```python
from build123d import *

# Parameters (mm, degrees)
SKETCH2_R           = 3.5
SKETCH2_R_2         = 1.5
BOSS_EXTRUDE1_DEPTH = 3.5
FILLET1_R           = 10
SKETCH3_R           = 1
CUT_EXTRUDE1_DEPTH  = 10


with BuildPart() as part:
    # Sketch2 → Boss-Extrude1 (new body)
    with BuildSketch(Plane.XY):
        with BuildLine():
            Line((-56.161165235, -8.838834765), (0, 47.32233047))
            Line((0, 47.32233047), (56.161165235, -8.838834765))
            ThreePointArc((56.161165235, -8.838834765), (73.838834765, -8.838834765), (73.838834765, 8.838834765))
            Line((73.838834765, 8.838834765), (0, 82.67766953))
            Line((0, 82.67766953), (-73.838834765, 8.838834765))
            ThreePointArc((-73.838834765, 8.838834765), (-73.838834765, -8.838834765), (-56.161165235, -8.838834765))
        make_face()
        with Locations((-65, 0)):
            Circle(SKETCH2_R, mode=Mode.SUBTRACT)
        with Locations((65, 0)):
            Circle(SKETCH2_R, mode=Mode.SUBTRACT)
        with Locations((0, 65)):
            Circle(SKETCH2_R_2, mode=Mode.SUBTRACT)
    extrude(amount=-BOSS_EXTRUDE1_DEPTH)

    # Fillet1
    fillet1_edges = [part.edges().sort_by_distance(p)[0] for p in [
        (0, 82.67766953, -1.75),
        (0, 47.32233047, -1.75),
    ]]
    fillet(fillet1_edges, radius=FILLET1_R)

    # Sketch3 → Cut-Extrude1 (cut)
    with BuildSketch(Plane.XY):
        with Locations((-52.625631329, 27.223611076)):
            Circle(SKETCH3_R)
        with Locations((-37.776388924, 12.374368671)):
            Circle(SKETCH3_R)
        with Locations((37.776388924, 12.374368671)):
            Circle(SKETCH3_R)
        with Locations((52.625631329, 27.223611076)):
            Circle(SKETCH3_R)
    extrude(amount=-CUT_EXTRUDE1_DEPTH, mode=Mode.SUBTRACT)


solid = part.part
```
Check sheet for the modelled part. Datum: model origin and axes. Units: mm. A direction names the side the tool comes from. Round coordinates to 2 decimals unless told otherwise and drop trailing zeros. Write each loop counter-clockwise with the first axis right and the second up, starting at its lowest first coordinate (ties: lowest second). Pieces come first, ordered by that corner, then holes. Notation, with made-up numbers: (31.25, 55) -> (64.25, 55) arc R9 cw to (64.25, 60) -> close; hole circle Ø3 at (-17, -14). An arc over 180 degrees is marked (long way). One line per question, with ' | ' between items. Start each with the question number.
1. Sectioned sample at C-C, the plane y = 0. Record the cut outline in (x, z), then the cut area to 3 significant figures.
2. Sectioned sample at A-A, the plane x = 0. Record the cut outline in (y, z), then the cut area to 3 significant figures.
3. Sectioned sample at D-D, the plane z = -2.5. Record the cut outline in (x, y), then the cut area to 3 significant figures.
4. Release check for a two-part mould opening along X. For faces 1 (the face through (11, 40, -3.5)), 2 (the face through (-0.11, 78.535, -1.774)), 3 (the face through (0.806, 66.265, -1.726)), 4 (the face through (-39.99, 42.69, -1.73)) record: +X half, -X half, draft (parallel to the pull), parting line (faces both ways), or undercut.
5. Scan lines: line 1 along X through (y, z) = (2, -2.8); line 2 along X through (y, z) = (-2, -2.45); line 3 along X through (y, z) = (19, -1). Record each from-to range of solid material in increasing order. Write a range as from..to.
6. Sectioned sample at B-B, the plane y = 65. Record the cut outline in (x, z), then the cut area to 3 significant figures.
7. Depth check by flat-ended pin: pin 1 (1 mm diameter, centred on y = 66, z = -2, fed in from +X); pin 2 (2 mm diameter, centred on y = 58.5, z = -1, fed in from +X); pin 3 (1.5 mm diameter, centred on y = 62, z = -0.5, fed in from +X). Enter the tip coordinate at first touch or a pass-through.
8. Set-up check for faces 5 (the face through (11, 40, 0)), 6 (the face through (-31.96, 15.36, -1.73)): record each of +Z, -Z, +X, -X, +Y, -Y from which the full face is reachable in a straight line by a thin tool's end or side.
Taken from the geometry:
1) outline: (-77.5, -3.5) -> (-68.5, -3.5) -> (-68.5, 0) -> (-77.5, 0) -> close; (-61.5, -3.5) -> (-47.32, -3.5) -> (-47.32, 0) -> (-61.5, 0) -> close; (47.32, -3.5) -> (61.5, -3.5) -> (61.5, 0) -> (47.32, 0) -> close; (68.5, -3.5) -> (77.5, -3.5) -> (77.5, 0) -> (68.5, 0) -> close | area: 162 mm^2
2) outline: (43.18, -3.5) -> (63.5, -3.5) -> (63.5, 0) -> (43.18, 0) -> close; (66.5, -3.5) -> (78.54, -3.5) -> (78.54, 0) -> (66.5, 0) -> close | area: 113 mm^2
3) outline: (-73.84, 8.84) arc R12.5 ccw to (-56.16, -8.84) -> (-7.07, 40.25) arc R10 cw to (7.07, 40.25) -> (56.16, -8.84) arc R12.5 ccw to (73.84, 8.84) -> (7.07, 75.61) arc R10 ccw to (-7.07, 75.61) -> close; hole circle Ø7 at (-65, 0); hole circle Ø2 at (-52.63, 27.22); hole circle Ø2 at (-37.78, 12.37); hole circle Ø3 at (0, 65); hole circle Ø2 at (37.78, 12.37); hole circle Ø2 at (52.63, 27.22); hole circle Ø7 at (65, 0) | area: 4,990 mm^2
4) face 1: draft | face 2: parting line | face 3: undercut | face 4: -X half
5) line 1: x = -77.34..-67.87, -62.13..-45.32, 45.32..62.13, 67.87..77.34 | line 2: x = -77.34..-67.87, -62.13..-49.32, 49.32..62.13, 67.87..77.34 | line 3: x = -63.68..-28.32, 28.32..63.68
6) outline: (-17.68, -3.5) -> (-1.5, -3.5) -> (-1.5, 0) -> (-17.68, 0) -> close; (1.5, -3.5) -> (17.68, -3.5) -> (17.68, 0) -> (1.5, 0) -> close | area: 113 mm^2
7) pin 1: stops at x = 17.18 | pin 2: stops at x = 25.18 | pin 3: stops at x = 21.43
8) face 5: +Z, +X, -X, +Y, -Y | face 6: +Z, -Z, -Y
